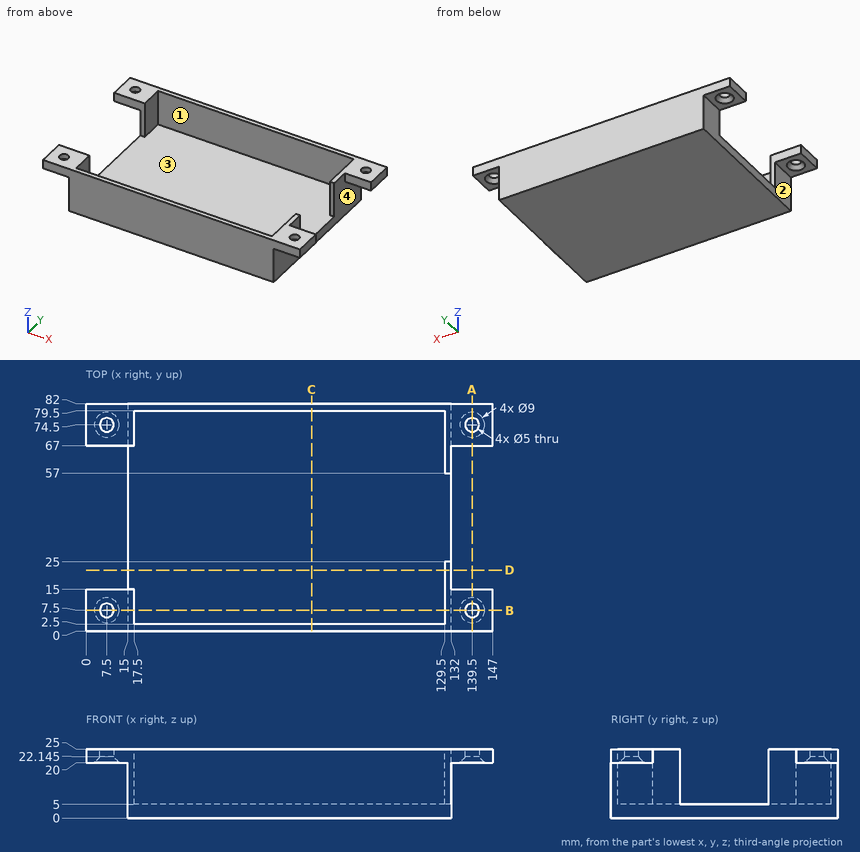
Answer from the drawing. Dimensions are ordinates in mm from the lowest x, y and z of the part. Give positions to 0.01 mm unless a question says otherwise; leave off trailing zeros. Order: outer loops, then holes, each group sorted by start corner. A loop starts at its lowest first (then second) coordinate and runs counter-clockwise, first axis right, second up.
(1) Find section D-D (y = 22). Give the vertices of the cut face in (x, z), plus the area to 3 significant figures.
(2) Given pin 1 (10 mm diameter, centred on y = 56.5, z = 8.5, fed in from -X); pin 2 (12 mm diameter, centred on x = 140, y = 6, fed in from -Z); pin 3 (6 mm diameter, centred on y = 8, z = 11.5, fed in from +X), each flat-ended and moving along its own axis, determine where each tip first touches the part or whether it passes through.
(3) Straight lines are drawn through the part: L1, parallel to Y at x = 139.5, z = 24.2; L2, parallel to Y at x = 89, z = 5.25; L3, parallel to Z at x = 45, y = 28.5. For each, find the intervals that lie inside material, in ascending order.
(4) Find section B-B (y = 7.5). Give the vertices of the cut face in (x, z) (1 decimal).
(5) For a pull along X with two mould halves and no side action, classify the marked faces 1, 2, 3 and 4 as released by +X, released by -X, zero draft, split by the parting line, or undercut.
(6) Find section A-A (x = 139.5). Give the vertices of the cut face in (y, z) (1 decimal).
(7) Find section C-C (x = 81.5). Give the vertices of the cut face in (y, z), plus the area to 3 significant figures.
Result sheet:
1. outline: (15, 0) - (132, 0) - (132, 25) - (129.5, 25) - (129.5, 5) - (15, 5) - close
1. area: 635 mm2
2. pin 1: stops at x = 15
2. pin 2: stops at z = 20
2. pin 3: stops at x = 132
3. L1: y = 0 to 5, 10 to 15, 67 to 72, 77 to 82
3. L2: y = 0 to 2.5, 79.5 to 82
3. L3: z = 0 to 5
4. outline: (0, 20) - (3, 20) - (5, 22.1) - (5, 25) - (0, 25) - close; (10, 22.1) - (12, 20) - (15, 20) - (15, 0) - (132, 0) - (132, 20) - (135, 20) - (137, 22.1) - (137, 25) - (129.5, 25) - (129.5, 5) - (17.5, 5) - (17.5, 25) - (10, 25) - close; (142, 22.1) - (144, 20) - (147, 20) - (147, 25) - (142, 25) - close
5. face 1: undercut
5. face 2: released by -X
5. face 3: undercut
5. face 4: released by +X
6. outline: (0, 20) - (3, 20) - (5, 22.1) - (5, 25) - (0, 25) - close; (10, 22.1) - (12, 20) - (15, 20) - (15, 25) - (10, 25) - close; (67, 20) - (70, 20) - (72, 22.1) - (72, 25) - (67, 25) - close; (77, 22.1) - (79, 20) - (82, 20) - (82, 25) - (77, 25) - close
7. outline: (0, 0) - (82, 0) - (82, 25) - (79.5, 25) - (79.5, 5) - (2.5, 5) - (2.5, 25) - (0, 25) - close
7. area: 510 mm2
